Can you work these out from the model? Positions are in its coordinate system, mm. A direction names the side the tool comes from. Give positions to 0.01 mm unless a question says otherwise; leave off trailing zeros. Loops run counter-clockwise (first coordinate to the right, second up) from the corner with the lowest first, then second, coordinate; pieces in that order, holes last. Notation, with made-up numbers: M -5,57.5 L 15,57.5 A24 ccw 15,78.5 Z; hole C -39,35.5 d7. An arc over 180 degrees is marked long. One line per item, written item: value. Start each with the question number.
from build123d import *

# Parameters (mm, degrees)
SKETCH1_W           = 76.2
SKETCH1_H           = 76.2
BOSS_EXTRUDE1_DEPTH = 3.175
SKETCH2_W           = 69.79412
SKETCH2_H           = 69.79412
SKETCH2_W_2         = 57.09412
SKETCH2_H_2         = 57.09412
BOSS_EXTRUDE2_DEPTH = 9.525
SKETCH13_R          = 4.7625
SKETCH13_W          = 25.4
SKETCH13_H          = 25.4
CUT_EXTRUDE1_DEPTH  = 3.175
SKETCH15_R          = 2.5527
CUT_EXTRUDE2_DEPTH  = 55.716959208
SKETCH17_R          = 4.7625
CUT_EXTRUDE3_DEPTH  = 6.35


with BuildPart() as part:
    # Sketch1 → Boss-Extrude1 (new body)
    with BuildSketch(Plane(origin=(0, 0, 0), x_dir=(1, 0, 0), z_dir=(0, 1, 0))):
        Rectangle(SKETCH1_W, SKETCH1_H)
    extrude(amount=BOSS_EXTRUDE1_DEPTH)

    # Sketch2 → Boss-Extrude2 (add)
    # profile 1 of 2: a face of its own
    with BuildSketch(Plane(origin=(0, 3.175, 0), x_dir=(1, 0, 0), z_dir=(0, 1, 0))):
        Rectangle(SKETCH2_W, SKETCH2_H)
        Rectangle(SKETCH2_W_2, SKETCH2_H_2, mode=Mode.SUBTRACT)
    # profile 2 of 2: a face of its own
    with BuildSketch(Plane(origin=(0, 3.175, 0), x_dir=(1, 0, 0), z_dir=(0, 1, 0))):
        Rectangle(SKETCH2_W_2, SKETCH2_H_2)
    extrude(amount=BOSS_EXTRUDE2_DEPTH)

    # Sketch9 → #6-32 Tapped Hole2 (revolve, cut)
    with BuildSketch(Plane(origin=(34.89706, 7.9375, 12.7), x_dir=(0, 0, -1), z_dir=(0, 1, 0))):
        Polygon((0, 0), (0, 11.98869403), (1.35255, 11.176), (1.35255, 0), align=None)
    f_6_32_tapped_hole2 = revolve(axis=Axis((41.24706, 7.9375, 12.7), (-1, 0, 0)), mode=Mode.SUBTRACT)

    # Mirror1: #6-32 Tapped Hole2 across plane
    add(f_6_32_tapped_hole2.mirror(Plane.XY), mode=Mode.SUBTRACT)

    # Mirror2: #6-32 Tapped Hole2 across plane
    add(f_6_32_tapped_hole2.mirror(Plane(origin=(0, 0, 0), x_dir=(0, 0, 1), z_dir=(1, 0, 0))), mode=Mode.SUBTRACT)

    # Mirror2 copy 1 sketch → Mirror2 copy 1 (revolve, cut)
    with BuildSketch(Plane(origin=(-34.89706, 7.9375, -12.7), x_dir=(0, 0, 1), z_dir=(0, 1, 0))):
        Polygon((0, 0), (0, 11.98869403), (1.35255, 11.176), (1.35255, 0), align=None)
    revolve(axis=Axis((-41.24706, 7.9375, -12.7), (1, 0, 0)), mode=Mode.SUBTRACT)

    # Sketch13 → Cut-Extrude1 (cut)
    with BuildSketch(Plane.XZ):
        with Locations((-12.7, -7.9375)):
            Circle(SKETCH13_R)
        with Locations((7.9375, -12.7)):
            Circle(SKETCH13_R)
        with Locations((12.7, 7.9375)):
            Circle(SKETCH13_R)
        with Locations((-7.9375, 12.7)):
            Circle(SKETCH13_R)
        Rectangle(SKETCH13_W, SKETCH13_H)
        with BuildLine():
            ThreePointArc((12.7, 12.7), (7.9375, 7.9375), (12.7, 3.175))
            Line((12.7, 3.175), (12.7, 12.7))
        make_face()
        with BuildLine():
            Line((12.7, 12.7), (12.7, 3.175))
            ThreePointArc((12.7, 3.175), (16.067596045, 4.569903955), (17.4625, 7.9375))
            ThreePointArc((17.4625, 7.9375), (16.067596045, 11.305096045), (12.7, 12.7))
        make_face()
        with BuildLine():
            ThreePointArc((-3.175, 12.7), (-7.9375, 17.4625), (-12.7, 12.7))
            Line((-12.7, 12.7), (-3.175, 12.7))
        make_face()
        with BuildLine():
            Line((-3.175, 12.7), (-12.7, 12.7))
            ThreePointArc((-12.7, 12.7), (-7.9375, 7.9375), (-3.175, 12.7))
        make_face()
        with BuildLine():
            ThreePointArc((-12.7, -3.175), (-17.4625, -7.9375), (-12.7, -12.7))
            Line((-12.7, -12.7), (-12.7, -3.175))
        make_face()
        with BuildLine():
            Line((-12.7, -3.175), (-12.7, -12.7))
            ThreePointArc((-12.7, -12.7), (-9.332403955, -11.305096045), (-7.9375, -7.9375))
            ThreePointArc((-7.9375, -7.9375), (-9.332403955, -4.569903955), (-12.7, -3.175))
        make_face()
        with BuildLine():
            ThreePointArc((12.7, -12.7), (7.9375, -7.9375), (3.175, -12.7))
            Line((3.175, -12.7), (12.7, -12.7))
        make_face()
        with BuildLine():
            Line((12.7, -12.7), (3.175, -12.7))
            ThreePointArc((3.175, -12.7), (7.9375, -17.4625), (12.7, -12.7))
        make_face()
    extrude(amount=-CUT_EXTRUDE1_DEPTH, mode=Mode.SUBTRACT)

    # Sketch15 → Cut-Extrude2 (cut, through all)
    with BuildSketch(Plane.XZ.offset(-3.175)):
        with Locations(Location((-6.35, 6.35, 0), (0, 0, 270))):
            Circle(SKETCH15_R)
        with Locations(Location((6.35, 6.35, 0), (0, 0, 270))):
            Circle(SKETCH15_R)
        with Locations(Location((6.35, -6.35, 0), (0, 0, 270))):
            Circle(SKETCH15_R)
        with Locations(Location((-6.35, -6.35, 0), (0, 0, 270))):
            Circle(SKETCH15_R)
    extrude(amount=-CUT_EXTRUDE2_DEPTH, mode=Mode.SUBTRACT)

    # Sketch17 → Cut-Extrude3 (cut)
    with BuildSketch(Plane(origin=(0, 12.7, 0), x_dir=(1, 0, 0), z_dir=(0, 1, 0))):
        with Locations(Location((-6.35, 6.35, 0), (0, 0, 270))):
            Circle(SKETCH17_R)
        with Locations(Location((6.35, 6.35, 0), (0, 0, 270))):
            Circle(SKETCH17_R)
        with Locations(Location((6.35, -6.35, 0), (0, 0, 270))):
            Circle(SKETCH17_R)
        with Locations(Location((-6.35, -6.35, 0), (0, 0, 270))):
            Circle(SKETCH17_R)
    extrude(amount=-CUT_EXTRUDE3_DEPTH, mode=Mode.SUBTRACT)


solid = part.part
Q1. If we section it at B-B, the plane z = 6.35: Give the number of separate pieces and of enclosed holes in the cut face, plus the area to 3 significant figures.
Q2. If we mould it in two halves opening along Y, with no side actions, what happens to faces 6 (the face through (29.4, 6.6, 12.9)), 7 (the face through (-23.05, 8.15, 12.59)), 8 (the face through (-34.897, 8, 0)), 9 (the face through (-1, 0, -17))? For each: released by +Y, released by -Y, zero draft, split by the parting line, or undercut.
Q3. Which directions (+Z, -Z, +X, -X, +Y, -Y) give clear straight access to the entire face, cutting with the end or side of a thin tool? Please do faces 1 (the face through (-12.7, 2, 5)), 2 (the face through (-3, 3.175, 37)), 3 (the face through (0, 8, 34.897)), 4 (the face through (-29.4, 6.6, -12.9)), 5 (the face through (29.4, 6.6, -12.9)).
Q4. I need wall thicknesses on line 1 along X through (y, z) = (10, 6.35); line 2 along Z through (x, y) = (-28, 8); line 3 along X through (y, z) = (5.5, 7). Which ranges of each line are inside material? Lowest first, please.
Q5. If we section it at D-D, the plane z = 20.5: Write out the boundary of the cut face in (x, y) (3 decimals).
Q6. If we section it at A-A, the plane y = 5: Write out the boundary of the cut face in (x, z).
Q7. For P1, Ø1.5, axis at y = 11, z = 14, coming from the +X side; P2, Ø4.5, axis at y = 7.94, z = 12.7, coming from the -X side; P3, Ø1.6, axis at y = 7.94, z = -12.7, coming from the -X side, each with a flat end and sliding along its axis, tell me the tip position at first contact or that it passes through.
Response:
1. separate pieces: 3
1. enclosed holes: 0
1. area: 658 mm^2
2. face 6: undercut
2. face 7: undercut
2. face 8: zero draft
2. face 9: released by -Y
3. face 1: -Y
3. face 2: +Y
3. face 3: +Z, +X, -X, +Y
3. face 4: -X
3. face 5: +X
4. line 1: -34.9 to -11.11, -1.59 to 1.59, 11.11 to 34.9
4. line 2: -34.9 to -14.05, -11.35 to 11.35, 14.05 to 34.9
4. line 3: -34.9 to -8.82, -3.88 to 3.88, 8.82 to 34.9
5. outline: M -38.1,0 L 38.1,0 L 38.1,3.175 L 34.897,3.175 L 34.897,12.7 L -34.897,12.7 L -34.897,3.175 L -38.1,3.175 Z
6. outline: M -34.9,-34.9 L 34.9,-34.9 L 34.9,34.9 L -34.9,34.9 Z; hole C -6.35,-6.35 d5.11; hole C -6.35,6.35 d5.11; hole C 6.35,-6.35 d5.11; hole C 6.35,6.35 d5.11
7. P1: x = 34.9
7. P2: x = -34.9
7. P3: x = -23.39
